Source: CAD feature listing. Evaluate the final solid. Frame: model axes, mm. A direction names the side the tool comes from. Coordinates: 2 decimals unless noted, no trailing zeros. Loops run counter-clockwise (first coordinate to the right, second up) from the corner with the lowest first, then second, coordinate; pieces in that order, holes last.
from build123d import *

# Parameters (mm, degrees)
SKETCH1_R           = 41.91
BOSS_EXTRUDE1_DEPTH = 4.7625
SKETCH2_R           = 8.89
BOSS_EXTRUDE2_DEPTH = 6.3246
CUT_EXTRUDE1_DEPTH  = 13.6492


with BuildPart() as part:
    # Sketch1 → Boss-Extrude1 (new body, symmetric)
    with BuildSketch(Plane(origin=(0, 0, 0), x_dir=(1, 0, 0), z_dir=(0, 1, 0))):
        Circle(SKETCH1_R)
    extrude(amount=BOSS_EXTRUDE1_DEPTH, both=True)

    # Sketch2 → Boss-Extrude2 (add, symmetric)
    with BuildSketch(Plane(origin=(0, 0, 0), x_dir=(1, 0, 0), z_dir=(0, 1, 0))):
        Circle(SKETCH2_R)
    extrude(amount=BOSS_EXTRUDE2_DEPTH, both=True)

    # Sketch3 → Cut-Extrude1 (cut, through all)
    with BuildSketch(Plane(origin=(0, 6.3246, 0), x_dir=(1, 0, 0), z_dir=(0, 1, 0))):
        Polygon((0, 7.376342509), (-6.3881, 3.688171255), (-6.3881, -3.688171255), (0, -7.376342509), (6.3881, -3.688171255), (6.3881, 3.688171255), align=None)
    extrude(amount=-CUT_EXTRUDE1_DEPTH, mode=Mode.SUBTRACT)


solid = part.part
Q1. Line query: line 1 along Y through (x, z) = (-14.5, 28); line 2 along X through (y, z) = (-0.5, -18); line 3 along X through (y, z) = (-4.25, -19). Output: solid intervals per line, ascending.
Q2. Section B-B, the plane y = -0.75. Return the cut outline in (x, z).
Q3. Contact query for flat-ended pins moving along their axis: pin 1 Ø1.5 at (x, y) = (18.5, 2) entering from +Z; pin 2 Ø10 at (x, z) = (2, -20.5) entering from -Y; pin 3 Ø3 at (x, y) = (20.5, 4) entering from +Z. Output: stop coordinate, or through.
Q4. Section D-D, the plane x = 28. Return the cut outline in (y, z), plus the area to 3 significant figures.
Q5. Section A-A, the plane z = 0. Return the cut outline in (x, y).
Q6. Section C-C, the plane x = -5. Return the cut outline in (y, z), plus the area to 3 significant figures.
Q7. Access query for faces 1 (the cylindrical face through (-1.93, -5.53, 8.68)), 2 (the cylindrical face through (-1.93, 5.55, 8.68)), 3 (the flat face through (3.239, 0.089, -5.506)). Directions: +Z, -Z, +X, -X, +Y, -Y. A direction counts if a zero-diameter tool reaches every point of the face in a straight line with its end or side. Return the directions, or none.
Q8. Draft query along Z for faces 4 (the flat face through (-1, -4.762, -10)), 5 (the cylindrical face through (-5.456, 0.067, -41.553)), 6 (the flat face through (-6.388, 0, 0)). Return one class per face: +Z half, -Z half, draft (parallel to the pull), parting line (faces both ways), or undercut.
Derived:
1. line 1: y = -4.76 to 4.76
1. line 2: x = -37.85 to 37.85
1. line 3: x = -37.36 to 37.36
2. outline: circle Ø83.82 at (0, 0); hole (-6.39, -3.69) - (0, -7.38) - (6.39, -3.69) - (6.39, 3.69) - (0, 7.38) - (-6.39, 3.69) - close
3. pin 1: stops at z = 37.97
3. pin 2: stops at y = -4.76
3. pin 3: stops at z = 37.36
4. outline: (-4.76, -31.18) - (4.76, -31.18) - (4.76, 31.18) - (-4.76, 31.18) - close
4. area: 594 mm2
5. outline: (-41.91, -4.76) - (-8.89, -4.76) - (-8.89, -6.32) - (-6.39, -6.32) - (-6.39, 6.32) - (-8.89, 6.32) - (-8.89, 4.76) - (-41.91, 4.76) - close; (6.39, -6.32) - (8.89, -6.32) - (8.89, -4.76) - (41.91, -4.76) - (41.91, 4.76) - (8.89, 4.76) - (8.89, 6.32) - (6.39, 6.32) - close
6. outline: (-6.32, -7.35) - (-4.76, -7.35) - (-4.76, -41.61) - (4.76, -41.61) - (4.76, -7.35) - (6.32, -7.35) - (6.32, -4.49) - (-6.32, -4.49) - close; (-6.32, 4.49) - (6.32, 4.49) - (6.32, 7.35) - (4.76, 7.35) - (4.76, 41.61) - (-4.76, 41.61) - (-4.76, 7.35) - (-6.32, 7.35) - close
6. area: 725 mm2
7. face 1: -Y
7. face 2: +Y
7. face 3: +Y, -Y
8. face 4: draft
8. face 5: parting line
8. face 6: undercut
